Can you work these out from the model? Positions are in its coordinate system, mm. A direction names the side the tool comes from. Coordinates: 2 decimals unless noted, no trailing zeros. Use a Markdown table: item, result. Add a question column.
(1) I want a section at A-A (x = 35). State how many separate pieces and enclosed holes the cut face has, and give its area (3 significant figures).
(2) On a 3-axis mill with a long thin cutter (end or side, diameter ignored), from which of +Z, -Z, +X, -X, +Y, -Y can I reach the whole of each face in a straight line? I mean faces 1 (the flat face through (14.126, 4.523, 14.158)), 2 (the cylindrical face through (13, 22, 37)), 3 (the cylindrical face through (9.86, 17.22, 40.495)), 4 (the cylindrical face through (34.785, 15.636, 36.409)), 5 (the flat face through (48, 29, 27)). Say none if no direction works.
(3) For pin 1 Ø1.5 at (x, y) = (20, 30.5) entering from -Z; pin 2 Ø1.6 at (y, z) = (28, 1.5) entering from +X; pin 3 Ø12 at (x, y) = (36, 4) entering from -Z, each with a flat end and sliding along its axis, tell me the tip position at first contact or that it passes through.
(4) We'd pull the mould along Z, two halves only. Please class faces 6 (the flat face through (47, 17, 0)), 7 (the cylindrical face through (18.16, 30.69, 5.94)), 8 (the flat face through (24.65, 28.11, 38.44)), 9 (the flat face through (20, 17, 36)): pulls with the +Z half, pulls with the -Z half, needs draft (parallel to the pull), parting line crosses it, or undercut.
(5) If I drill on L1, parallel to Y at x = 35, z = 28.1; L2, parallel to X at y = 6.5, z = 30; L3, parallel to Z at x = 6, y = 4.5, over which ranges is the centre line in solid material (lowest first)? Write a range as [from, to].
```python
from build123d import *

# Parameters (mm, degrees)
CYLINDER023_R               = 1.5
CYLINDER023_DEPTH           = 48
CYLINDER022_R               = 1.5
CYLINDER022_DEPTH           = 48
CYLINDER021_R               = 1.65
CYLINDER021_DEPTH           = 20
CYLINDER021_PLACEMENT_ANGLE = 45
CYLINDER020_R               = 1.65
CYLINDER020_DEPTH           = 20
CYLINDER020_PLACEMENT_ANGLE = 45
BOX008_W                    = 10
BOX008_H                    = 34
BOX008_DEPTH                = 10
BOX008_PLACEMENT_ANGLE      = 45
CYLINDER018_R               = 5
CYLINDER018_DEPTH           = 20
CYLINDER019_R               = 5
CYLINDER019_DEPTH           = 20
CYLINDER017_R               = 5
CYLINDER017_DEPTH           = 38
BOX006_W                    = 15
BOX006_H                    = 34
BOX006_DEPTH                = 2
CYLINDER011_R               = 2.5
CYLINDER011_DEPTH           = 10
CYLINDER012_R               = 2.5
CYLINDER012_DEPTH           = 10
CYLINDER009_R               = 1.65
CYLINDER009_DEPTH           = 34
CYLINDER010_R               = 1.65
CYLINDER010_DEPTH           = 34
CYLINDER008_R               = 1.65
CYLINDER008_DEPTH           = 34
CYLINDER001_R               = 9
CYLINDER001_DEPTH           = 26
CYLINDER_R                  = 30.5
CYLINDER_DEPTH              = 26
BOX002_W                    = 72
BOX002_H                    = 20
BOX002_DEPTH                = 50
BOX002_PLACEMENT_ANGLE      = 53
BOX003_W                    = 72
BOX003_H                    = 20
BOX003_DEPTH                = 50
BOX003_PLACEMENT_ANGLE      = 53
COMPOUND_PLACEMENT_ANGLE    = 180
BOX001_W                    = 100
BOX001_H                    = 34
BOX001_DEPTH                = 50
BOX001_PLACEMENT_ANGLE      = 45
BOX_W                       = 50
BOX_H                       = 34
BOX_DEPTH                   = 43


with BuildPart() as cylinder023:
    # Cylinder023 → Cylinder023 (new body)
    with BuildSketch(Plane(origin=(0, 29, 26), x_dir=(0, 0, -1), z_dir=(1, 0, 0))):
        Circle(CYLINDER023_R)
    extrude(amount=CYLINDER023_DEPTH)


with BuildPart() as cabledrillhole:
    # Cylinder022 → Cylinder022 (new body)
    with BuildSketch(Plane(origin=(0, 5, 26), x_dir=(0, 0, -1), z_dir=(1, 0, 0))):
        Circle(CYLINDER022_R)
    extrude(amount=CYLINDER022_DEPTH)

    # Fusion008: union Cylinder023
    add(cylinder023.part)


with BuildPart() as cylinder021:
    # Cylinder021 → Cylinder021 (new body)
    with BuildSketch(Plane.XY):
        Circle(CYLINDER021_R)
    extrude(amount=CYLINDER021_DEPTH)


with BuildPart() as cylinder021_1:
    # Cylinder021 placement: moved
    add(cylinder021.part.moved(Location((0, 29.5, 0))).rotate(Axis((0, 29.5, 0), (0, 1, 0)), CYLINDER021_PLACEMENT_ANGLE))


with BuildPart() as m4screws:
    # Cylinder020 → Cylinder020 (new body)
    with BuildSketch(Plane.XY):
        Circle(CYLINDER020_R)
    extrude(amount=CYLINDER020_DEPTH)


with BuildPart() as m4screws_1:
    # Cylinder020 placement: moved
    add(m4screws.part.moved(Location((0, 4.5, 0))).rotate(Axis((0, 4.5, 0), (0, 1, 0)), CYLINDER020_PLACEMENT_ANGLE))

    # Fusion007: union Cylinder021
    add(cylinder021_1.part)


with BuildPart() as cube008:
    # Box008 → Box008 (new body)
    with BuildSketch(Plane.XY):
        with Locations((5, 17)):
            Rectangle(BOX008_W, BOX008_H)
    extrude(amount=BOX008_DEPTH)


with BuildPart() as cube008_1:
    # Box008 placement: moved
    add(cube008.part.moved(Location((-7, 0, 0))).rotate(Axis((-7, 0, 0), (0, 1, 0)), BOX008_PLACEMENT_ANGLE))


with BuildPart() as nitrogenchamber002:
    # Cylinder018 → Cylinder018 (new body)
    with BuildSketch(Plane(origin=(0, 17, 14.5), x_dir=(0, 0, -1), z_dir=(1, 0, 0))):
        Circle(CYLINDER018_R)
    extrude(amount=CYLINDER018_DEPTH)


with BuildPart() as nitrogenchamber003:
    # Cylinder019 → Cylinder019 (new body)
    with BuildSketch(Plane(origin=(0, 17, 35.5), x_dir=(0, 0, -1), z_dir=(1, 0, 0))):
        Circle(CYLINDER019_R)
    extrude(amount=CYLINDER019_DEPTH)


with BuildPart() as nitrogenchamber:
    # Cylinder017 → Cylinder017 (new body)
    with BuildSketch(Plane(origin=(13, 17, 0), x_dir=(0, 1, 0), z_dir=(0, 0, 1))):
        Circle(CYLINDER017_R)
    extrude(amount=CYLINDER017_DEPTH)

    # Fusion006: union NitrogenChamber002, NitrogenChamber003
    add(nitrogenchamber002.part)
    add(nitrogenchamber003.part)


with BuildPart() as cube006:
    # Box006 → Box006 (new body)
    with BuildSketch(Plane(origin=(15, 0, 0), x_dir=(1, 0, 0), z_dir=(0, 0, 1))):
        with Locations((7.5, 17)):
            Rectangle(BOX006_W, BOX006_H)
    extrude(amount=BOX006_DEPTH)


with BuildPart() as cylinder011:
    # Cylinder011 → Cylinder011 (new body)
    with BuildSketch(Plane(origin=(20, 5, 0), x_dir=(1, 0, 0), z_dir=(0, 0, 1))):
        Circle(CYLINDER011_R)
    extrude(amount=CYLINDER011_DEPTH)


with BuildPart() as obj1:
    # Cylinder012 → Cylinder012 (new body)
    with BuildSketch(Plane(origin=(20, 29, 0), x_dir=(1, 0, 0), z_dir=(0, 0, 1))):
        Circle(CYLINDER012_R)
    extrude(amount=CYLINDER012_DEPTH)

    # Fusion002: union Cylinder011
    add(cylinder011.part)


with BuildPart() as cylinder009:
    # Cylinder009 → Cylinder009 (new body)
    with BuildSketch(Plane(origin=(35, 20, 27), x_dir=(1, 0, 0), z_dir=(0, 0, 1))):
        Circle(CYLINDER009_R)
    extrude(amount=CYLINDER009_DEPTH)


with BuildPart() as cylinder010:
    # Cylinder010 → Cylinder010 (new body)
    with BuildSketch(Plane(origin=(35, 14, 27), x_dir=(1, 0, 0), z_dir=(0, 0, 1))):
        Circle(CYLINDER010_R)
    extrude(amount=CYLINDER010_DEPTH)


with BuildPart() as m4mountscrews01_corehole:
    # Cylinder008 → Cylinder008 (new body)
    with BuildSketch(Plane(origin=(35, 34, 30), x_dir=(1, 0, 0), z_dir=(0, -1, 0))):
        Circle(CYLINDER008_R)
    extrude(amount=CYLINDER008_DEPTH)

    # Fusion001: union Cylinder009, Cylinder010
    add(cylinder009.part)
    add(cylinder010.part)


with BuildPart() as cylinder001:
    # Cylinder001 → Cylinder001 (new body)
    with BuildSketch(Plane.XY):
        Circle(CYLINDER001_R)
    extrude(amount=CYLINDER001_DEPTH)


with BuildPart() as cut001:
    # Cylinder → Cylinder (new body)
    with BuildSketch(Plane.XY):
        Circle(CYLINDER_R)
    extrude(amount=CYLINDER_DEPTH)

    # Cut001: cut Cylinder001
    add(cylinder001.part, mode=Mode.SUBTRACT)


with BuildPart() as cut001_1:
    # Cut001 placement: moved
    add(cut001.part.moved(Location((51.5, 17, 0))))


with BuildPart() as cube002:
    # Box002 → Box002 (new body)
    with BuildSketch(Plane.XY):
        with Locations((36, 10)):
            Rectangle(BOX002_W, BOX002_H)
    extrude(amount=BOX002_DEPTH)


with BuildPart() as cube002_1:
    # Box002 placement: moved
    add(cube002.part.moved(Location((0, 34, 34))).rotate(Axis((0, 34, 34), (1, 0, 0)), BOX002_PLACEMENT_ANGLE))


with BuildPart() as compound:
    # Box003 → Box003 (new body)
    with BuildSketch(Plane.XY):
        with Locations((36, 10)):
            Rectangle(BOX003_W, BOX003_H)
    extrude(amount=BOX003_DEPTH)


with BuildPart() as compound_1:
    # Box003 placement: moved
    add(compound.part.moved(Location((0, 34, 34))).rotate(Axis((0, 34, 34), (1, 0, 0)), BOX003_PLACEMENT_ANGLE))


with BuildPart() as compound_2:
    # Compound placement: moved
    add(compound_1.part.moved(Location((72, 34, 0))).rotate(Axis((72, 34, 0), (0, 0, 1)), COMPOUND_PLACEMENT_ANGLE))


with BuildPart() as fusion:
    # Box001 → Box001 (new body)
    with BuildSketch(Plane.XY):
        with Locations((50, 17)):
            Rectangle(BOX001_W, BOX001_H)
    extrude(amount=BOX001_DEPTH)


with BuildPart() as fusion_1:
    # Box001 placement: moved
    add(fusion.part.moved(Location((41, 0, 43))).rotate(Axis((41, 0, 43), (0, 1, 0)), BOX001_PLACEMENT_ANGLE))

    # Fusion: union Cube002, Compound
    add(cube002_1.part)
    add(compound_2.part)


with BuildPart() as obj2:
    # Box → Box (new body)
    with BuildSketch(Plane.XY):
        with Locations((25, 17)):
            Rectangle(BOX_W, BOX_H)
    extrude(amount=BOX_DEPTH)

    # Cut: cut Fusion
    add(fusion_1.part, mode=Mode.SUBTRACT)

    # Cut003: cut Cut001
    add(cut001_1.part, mode=Mode.SUBTRACT)

    # Cut008: cut M4Mountscrews01_Corehole
    add(m4mountscrews01_corehole.part, mode=Mode.SUBTRACT)

    # Cut009: cut obj1
    add(obj1.part, mode=Mode.SUBTRACT)

    # Cut011: cut Cube006
    add(cube006.part, mode=Mode.SUBTRACT)

    # Cut014: cut NitrogenChamber
    add(nitrogenchamber.part, mode=Mode.SUBTRACT)

    # Cut015: cut Cube008
    add(cube008_1.part, mode=Mode.SUBTRACT)

    # Cut016: cut M4Screws
    add(m4screws_1.part, mode=Mode.SUBTRACT)

    # Cut017: cut CableDrillHole
    add(cabledrillhole.part, mode=Mode.SUBTRACT)


solid = obj2.part
```
Answers follow:
| question | item | result |
|---|---|---|
| 1 | separate pieces | 4 |
| 1 | enclosed holes | 0 |
| 1 | area | 267 mm² |
| 2 | face 1 | none |
| 2 | face 2 | -Z |
| 2 | face 3 | -X |
| 2 | face 4 | +Z |
| 2 | face 5 | -Z, -X |
| 3 | pin 1 | stops at z = 10 |
| 3 | pin 2 | stops at x = 23.3 |
| 3 | pin 3 | stops at z = 26 |
| 4 | face 6 | pulls with the -Z half |
| 4 | face 7 | needs draft |
| 4 | face 8 | pulls with the +Z half |
| 4 | face 9 | undercut |
| 5 | L1 | y = [0, 12.35], [15.65, 18.35], [21.65, 34] |
| 5 | L2 | x = [0, 33.35], [36.65, 50] |
| 5 | L3 | z = [1.14, 3.67], [8.33, 24.59], [27.41, 37.39] |
